Input: part model. Units: mm. Frame: model coordinates. A direction names the side the tool comes from. Give positions to 0.01 mm unless a question says otherwise; leave off trailing zeros. Loops run counter-clockwise (first coordinate to the right, second up) from the corner with the lowest first, then second, coordinate; pieces in that order, holes last. Notation, with made-up numbers: (-30.75, 21) -> (15.25, 21) arc R22 ccw to (15.25, 38) -> close; hole circle Ø4 at (49, 78.5). An arc over 180 degrees is marked (long way). Answer as a JSON object with one key per item and string values. Group by question number.
```python
from build123d import *

# Parameters (mm, degrees)
FILLET3_R          = 5
SKETCH2_R          = 6
CUT_EXTRUDE1_DEPTH = 68
CIRPATTERN1_COUNT  = 5


with BuildPart() as part:
    # Sketch1 → Revolve1 (revolve)
    with BuildSketch(Plane.XY):
        Polygon((0, 130), (0, 85.73), (-12.7, 85.73), (-12.7, 78.25), (-40, 78.25), (-40, 88.25), (-25, 88.25), (-25, 164), (43, 164), (43, 140), (53, 140), (53, 130), align=None)
    revolve(axis=Axis((100.288511214, 0, 0), (-1, 0, 0)))

    # Fillet3
    fillet3_edges = [part.edges().sort_by_distance(p)[0] for p in [
        (-25, -88.25, 0),
    ]]
    fillet(fillet3_edges, radius=FILLET3_R)

    # Sketch2 → Cut-Extrude1 (cut)
    with BuildSketch(Plane(origin=(43, 0, 0), x_dir=(0, 0, -1), z_dir=(1, 0, 0))):
        with Locations((0, 152)):
            Circle(SKETCH2_R)
    cut_extrude1 = extrude(amount=-CUT_EXTRUDE1_DEPTH, mode=Mode.SUBTRACT)

    # CirPattern1: Cut-Extrude1 ×5 about axis
    cirpattern1_axis = Axis((0, 0, 0), (1, 0, 0))
    for i in range(1, CIRPATTERN1_COUNT):
        add(cut_extrude1.rotate(cirpattern1_axis, i * 360 / CIRPATTERN1_COUNT), mode=Mode.SUBTRACT)


solid = part.part
```
Q1. Ray query, probe 1 along Y at (x, z) = (11, 0); probe 2 along Z at (x, y) = (-4.5, 0); probe 3 along Z at (x, y) = (-32, 0). Return the intervals inside material, ascending.
Q2. Section D-D on y = 0. Return the cut outline in (x, z).
Q3. Pull-direction query (Z, two-part tool) for faces 1 (the face through (0, 85, 27)), 2 (the face through (9, -36, 160)), 3 (the face through (53, 124, 41)); classes: +Z half, -Z half, draft (parallel to the pull), parting line (faces both ways), or undercut.
Q4. Set-up query: faces 4 (the face through (-34.93, -70.03, 53.7)), 5 (the face through (9.476, 146.143, 1.301)), 6 (the face through (48.07, -111.1, 85.19)). Return all of +Z, -Z, +X, -X, +Y, -Y with unobstructed straight access to the full face (end or side cutting, diameter ignored); none if empty.
Q5. Section C-C on x = 32. Return the cut outline in (y, z), then the cut area to 3 significant figures.
Q6. Pin query (flat end, axial travel): pin 1 Ø3 at (x, z) = (32.5, -50) entering from -Y; pin 2 Ø8 at (x, z) = (32.5, -55) entering from -Y; pin 3 Ø14 at (y, z) = (152, 0) entering from -X; pin 4 Ø4 at (y, z) = (-12, -127.5) entering from +X. Return the tip coordinate at first contact, or that it passes through.
Q7. Section B-B on y = 152. Return the cut outline in (x, z), then the cut area to 3 significant figures.
Q8. Section A-A on z = 0. State how many separate pieces and enclosed holes the cut face has, then the cut area to 3 significant figures.
Numbers:
{
 "1": {"probe 1": "y = -164 to -130, 130 to 146, 158 to 164", "probe 2": "z = -164 to -85.73, 85.73 to 164", "probe 3": "z = -88.25 to -78.25, 78.25 to 88.25"},
 "2": {"outline": "(-40, -88.25) -> (-30, -88.25) arc R5 cw to (-25, -93.25) -> (-25, -164) -> (43, -164) -> (43, -140) -> (53, -140) -> (53, -130) -> (0, -130) -> (0, -85.73) -> (-12.7, -85.73) -> (-12.7, -78.25) -> (-40, -78.25) -> close; (-40, 78.25) -> (-12.7, 78.25) -> (-12.7, 85.73) -> (0, 85.73) -> (0, 130) -> (53, 130) -> (53, 140) -> (43, 140) -> (43, 164) -> (-25, 164) -> (-25, 93.25) arc R5 cw to (-30, 88.25) -> (-40, 88.25) -> close"},
 "3": {"face 1": "undercut", "face 2": "parting line", "face 3": "draft"},
 "4": {"face 4": "-X", "face 5": "+X, -X", "face 6": "+X"},
 "5": {"outline": "circle Ø328 at (0, 0); hole circle Ø260 at (0, 0); hole circle Ø12 at (-122.97, -89.34); hole circle Ø12 at (-122.97, 89.34); hole circle Ø12 at (46.97, -144.56); hole circle Ø12 at (46.97, 144.56); hole circle Ø12 at (152, 0)", "area": "30,800 mm²"},
 "6": {"pin 1": "stops at y = -156.66", "pin 2": "stops at y = -155.87", "pin 3": "stops at x = -25", "pin 4": "stops at x = 53"},
 "7": {"outline": "(-25, -61.58) -> (43, -61.58) -> (43, -6) -> (-25, -6) -> close; (-25, 6) -> (43, 6) -> (43, 61.58) -> (-25, 61.58) -> close", "area": "7,560 mm²"},
 "8": {"separate pieces": "3", "enclosed holes": "0", "area": "6,720 mm²"}
}
